Input: part model. Units: mm. Frame: model coordinates. Face numbers are marked on the shaded views. A direction names the side the tool comes from. Give positions to 0.01 mm unless a question says otherwise; leave off trailing zeros. Loops run counter-clockwise (first coordinate to the right, second up) from the corner with the lowest first, then second, coordinate; pieces in that order, holes last. Notation, with made-up numbers: (62.5, -37.75) -> (79.5, -37.75) arc R14 cw to (79.5, -28.75) -> close; hole circle Ø6 at (12.25, 75). An arc over 180 degrees is marked (long way). Answer as a JSON object with one key per item and string values.
```python
from build123d import *

# Parameters (mm, degrees)
CUT_EXTRUDE1_DEPTH = 3.25


with BuildPart() as part:
    # Sketch1 → Revolve3 (revolve)
    with BuildSketch(Plane(origin=(0, 0, 0), x_dir=(1, 0, 0), z_dir=(0, 1, 0)), mode=Mode.PRIVATE) as revolve3_sk:
        with BuildLine():
            Line((-25.676880223, 0), (44.323119777, 0))
            Line((44.323119777, 0), (44.323119777, 12.5))
            Line((44.323119777, 12.5), (-5.676880223, 12.5))
            Line((-5.676880223, 12.5), (-5.676880223, 17))
            ThreePointArc((-5.676880223, 17), (-7.141346317, 20.535533906), (-10.676880223, 22))
            Line((-10.676880223, 22), (-86.676880223, 22))
            Line((-86.676880223, 22), (-86.676880223, 31.774373259))
            ThreePointArc((-86.676880223, 31.774373259), (-88.141346317, 35.309907165), (-91.676880223, 36.774373259))
            Line((-91.676880223, 36.774373259), (-106.676880223, 36.774373259))
            ThreePointArc((-106.676880223, 36.774373259), (-110.212414129, 35.309907165), (-111.676880223, 31.774373259))
            Line((-111.676880223, 31.774373259), (-111.676880223, 21))
            ThreePointArc((-111.676880223, 21), (-110.212414129, 17.464466094), (-106.676880223, 16))
            Line((-106.676880223, 16), (-25.676880223, 16))
            Line((-25.676880223, 16), (-25.676880223, 0))
        make_face()
    revolve(revolve3_sk.sketch.rotate(Axis((-25.676880223, 0, 0), (1, 0, 0)), 180), axis=Axis((-25.676880223, 0, 0), (1, 0, 0)))

    # Sketch3 → Cut-Extrude1 (cut, symmetric)
    with BuildSketch(Plane.XY):
        Polygon((-86.676880223, 0), (-86.676880223, 50), (-51.676880223, 50), (-59.676880223, -56.407142019), (-86.676880223, -56.407142019), align=None)
    extrude(amount=CUT_EXTRUDE1_DEPTH, both=True, mode=Mode.SUBTRACT)


solid = part.part
```
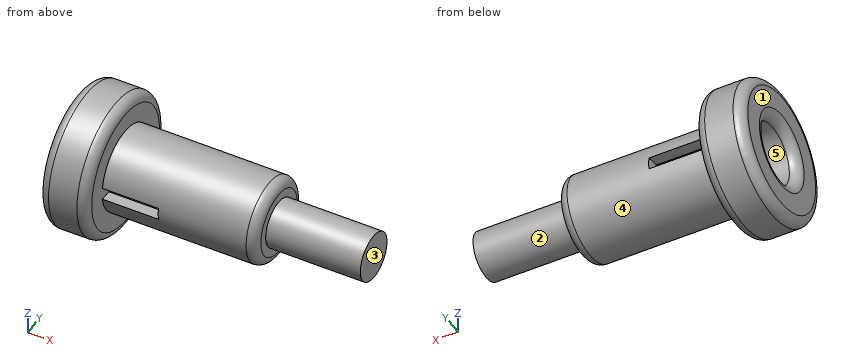
Q1. Section D-D, the plane x = -40. Return the cut outline in (y, z), then the cut area to 3 significant figures.
Evaluation:
{"outline": "circle Ø44 at (0, 0); hole circle Ø32 at (0, 0)", "area": "716 mm2"}
Q2. Access query for the marked faces 1 and 2. Directions: +Z, -Z, +X, -X, +Y, -Y. A direction counts if a zero-diameter tool reaches every point of the face in a straight line with its end or side. Return the directions, or none.
Evaluation:
{"face 1": "+Z, -Z, -X, +Y, -Y", "face 2": "+X"}
Q3. Draft query along Z for the marked faces 3, 4 and 5. Return one class per face: +Z half, -Z half, draft (parallel to the pull), parting line (faces both ways), or undercut.
Evaluation:
{"face 3": "draft", "face 4": "parting line", "face 5": "undercut"}
Q4. Pin query (flat end, axial travel): pin 1 (1.8 mm diameter, centred on x = -69.5, y = 17.5, fed in from -Z); pin 2 (1 mm diameter, centred on x = -28, y = 8.5, fed in from +Z); pin 3 (6.5 mm diameter, centred on x = -69.5, y = -17.5, fed in from +Z). Return the tip coordinate at first contact, or that it passes through.
Evaluation:
{"pin 1": "stops at z = -14.44", "pin 2": "stops at z = 20.49", "pin 3": "stops at z = 16.76"}
Q5. Ray query, line 1 along X through (y, z) = (11, 27.5); line 2 along X through (y, z) = (-3.5, 12.5); line 3 along Y through (x, z) = (-44.5, 0). Return the intervals inside material, ascending.
Evaluation:
{"line 1": "x = -111.68 to -86.68", "line 2": "x = -25.68 to -5.68", "line 3": "y = -22 to -16, 16 to 22"}
Q6. Section B-B, the plane y = 0. Return the cut outline in (x, z).
Evaluation:
{"outline": "(-111.68, -31.77) arc R5 ccw to (-106.68, -36.77) -> (-91.68, -36.77) arc R5 ccw to (-86.68, -31.77) -> (-86.68, -22) -> (-10.68, -22) arc R5 ccw to (-5.68, -17) -> (-5.68, -12.5) -> (44.32, -12.5) -> (44.32, 12.5) -> (-5.68, 12.5) -> (-5.68, 17) arc R5 ccw to (-10.68, 22) -> (-86.68, 22) -> (-86.68, 31.77) arc R5 ccw to (-91.68, 36.77) -> (-106.68, 36.77) arc R5 ccw to (-111.68, 31.77) -> (-111.68, 21) arc R5 ccw to (-106.68, 16) -> (-25.68, 16) -> (-25.68, -16) -> (-106.68, -16) arc R5 ccw to (-111.68, -21) -> close"}
Q7. Section A-A, the plane x = -76. Return the cut outline in (y, z), then the cut area to 3 significant figures.
Evaluation:
{"outline": "(-21.76, -3.25) arc R22 ccw to (21.76, -3.25) -> (15.67, -3.25) arc R16 cw to (-15.67, -3.25) -> close; (-21.76, 3.25) -> (-15.67, 3.25) arc R16 cw to (15.67, 3.25) -> (21.76, 3.25) arc R22 ccw to start", "area": "638 mm2"}
Q8. Section C-C, the plane z = 0. Return the cut outline in (x, y), then the cut area to 3 significant figures.
Evaluation:
{"outline": "(-111.68, -31.77) arc R5 ccw to (-106.68, -36.77) -> (-91.68, -36.77) arc R5 ccw to (-86.68, -31.77) -> (-86.68, -16) -> (-106.68, -16) arc R5 ccw to (-111.68, -21) -> close; (-111.68, 21) arc R5 ccw to (-106.68, 16) -> (-86.68, 16) -> (-86.68, 31.77) arc R5 ccw to (-91.68, 36.77) -> (-106.68, 36.77) arc R5 ccw to (-111.68, 31.77) -> close; (-57.09, -22) -> (-10.68, -22) arc R5 ccw to (-5.68, -17) -> (-5.68, -12.5) -> (44.32, -12.5) -> (44.32, 12.5) -> (-5.68, 12.5) -> (-5.68, 17) arc R5 ccw to (-10.68, 22) -> (-53.78, 22) -> (-54.23, 16) -> (-25.68, 16) -> (-25.68, -16) -> (-56.64, -16) -> close", "area": "3,480 mm2"}
